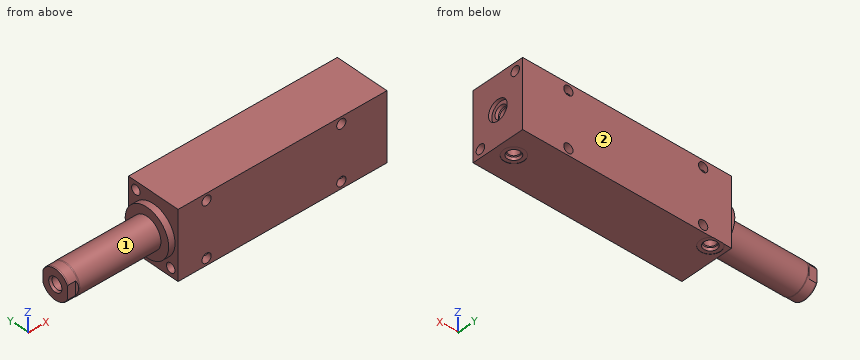
from build123d import *

# Parameters (mm, degrees)
SKETCH1_W          = 63.5
SKETCH1_H          = 50.8
EXTRUDE1_DEPTH     = 196.85
SKETCH5_R          = 22.225
EXTRUDE2_DEPTH     = 5.969
SKETCH6_W          = 14.2875
SKETCH6_H          = 86.36
CUT_EXTRUDE4_DEPTH = 30.48
HOLE1_D            = 8.7376
HOLE1_DEPTH        = 196.85
HOLE2_D            = 8.7376
HOLE2_DEPTH        = 50.8
LPATTERN1_COUNT    = 2
LPATTERN1_PITCH    = 127


with BuildPart() as part:
    # Sketch1 → Extrude1 (new body)
    with BuildSketch(Plane(origin=(0, 0, 0), x_dir=(0, 0, -1), z_dir=(1, 0, 0))):
        Rectangle(SKETCH1_W, SKETCH1_H)
    extrude(amount=EXTRUDE1_DEPTH)

    # S2D0002 → Cut-Revolve1 (revolve, cut)
    with BuildSketch(Plane(origin=(0, 17.4752, 0), x_dir=(-1, 0, 0), z_dir=(0, 1, 0)), mode=Mode.PRIVATE) as cut_revolve1_sk:
        Polygon((-18.8849, -31.496), (-22.225, -31.496), (-22.225, -31.75), (-12.7, -31.75), (-12.7, -17.526), (-17.6784, -17.526), (-17.6784, -28.279393135), (-18.342306865, -28.9433), align=None)
    revolve(cut_revolve1_sk.sketch.rotate(Axis((12.7, 17.4752, -19.13842003), (0, 0, 1)), 180), axis=Axis((12.7, 17.4752, -19.13842003), (0, 0, 1)), mode=Mode.SUBTRACT)  # turned: the seam where the file's is

    # Sketch3 → Cut-Revolve2 (revolve, cut)
    with BuildSketch(Plane(origin=(41.148, 0, -25.146), x_dir=(1, 0, 0), z_dir=(0, 1, 0))):
        Polygon((146.7993, 6.35), (150.1394, 6.35), (150.1394, 6.604), (140.6144, 6.604), (140.6144, -7.62), (145.5928, -7.62), (145.5928, 3.133393135), (146.256706865, 3.7973), align=None)
    revolve(axis=Axis((181.7624, 0, -3.189624441), (0, 0, -1)), mode=Mode.SUBTRACT)

    # Sketch4 → Cut-Revolve3 (revolve, cut)
    with BuildSketch(Plane(origin=(53.975, 0, 0), x_dir=(0, -1, 0), z_dir=(0, 0, 1)), mode=Mode.PRIVATE) as cut_revolve3_sk:
        Polygon((6.1849, 139.827), (9.525, 139.827), (9.525, 142.875), (0, 142.875), (0, 128.4732), (4.9784, 128.4732), (4.9784, 136.610393135), (5.642306865, 137.2743), align=None)
    revolve(cut_revolve3_sk.sketch.rotate(Axis((38.879609832, 0, 0), (1, 0, 0)), 270), axis=Axis((38.879609832, 0, 0), (1, 0, 0)), mode=Mode.SUBTRACT)  # turned: the seam where the file's is

    # Sketch5 → Extrude2 (add)
    with BuildSketch(Plane.ZY):
        Circle(SKETCH5_R)
    extrude(amount=EXTRUDE2_DEPTH)

    # Sketch6 → Revolve1 (revolve)
    with BuildSketch(Plane(origin=(0, 0, 0), x_dir=(0, 0, 1), z_dir=(0, -1, 0)), mode=Mode.PRIVATE) as revolve1_sk:
        with Locations((-7.14375, 49.149)):
            Rectangle(SKETCH6_W, SKETCH6_H)
    revolve(revolve1_sk.sketch.rotate(Axis((5.754582971, 0, 0), (-1, 0, 0)), 180), axis=Axis((5.754582971, 0, 0), (-1, 0, 0)))  # turned: the seam where the file's is

    # S2D0001 → Cut-Revolve4 (revolve, cut)
    with BuildSketch(Plane(origin=(-18.511260017, 3.2639, 0), x_dir=(0, 1, 0), z_dir=(0, 0, 1)), mode=Mode.PRIVATE) as cut_revolve4_sk:
        Polygon((2.286, 71.750017728), (2.286, 57.434739983), (-3.2639, 57.434739983), (-3.2639, 73.817739983), (3.4798, 73.817739983), align=None)
    revolve(cut_revolve4_sk.sketch.rotate(Axis((0, 0, 0), (-1, 0, 0)), 270), axis=Axis((0, 0, 0), (-1, 0, 0)), mode=Mode.SUBTRACT)  # turned: the seam where the file's is

    # Sketch8 → Cut-Revolve5 (revolve, cut)
    with BuildSketch(Plane(origin=(0, 0, 0), x_dir=(0, 0, -1), z_dir=(0, 1, 0)), mode=Mode.PRIVATE) as cut_revolve5_sk:
        with BuildLine():
            Line((-14.2875, 82.423), (-14.097, 83.185))
            Line((-14.097, 83.185), (-14.097, 91.313))
            ThreePointArc((-14.097, 91.313), (-13.996678675, 91.856796865), (-13.708922533, 92.329))
            Line((-13.708922533, 92.329), (-14.2875, 92.329))
            Line((-14.2875, 92.329), (-14.2875, 82.423))
        make_face()
    revolve(cut_revolve5_sk.sketch.rotate(Axis((-12.65936, 0, 0), (-1, 0, 0)), 180), axis=Axis((-12.65936, 0, 0), (-1, 0, 0)), mode=Mode.SUBTRACT)  # turned: the seam where the file's is

    # Sketch12 → Cut-Extrude4 (cut, symmetric)
    with BuildSketch(Plane(origin=(0, 0, 0), x_dir=(0, -1, 0), z_dir=(0, 0, -1))):
        Polygon((12.573, 92.329), (12.573, 84.7598), (14.097, 83.2358), (14.097, 92.329), align=None)
        Polygon((-12.573, 92.329), (-12.573, 84.7598), (-14.097, 83.2358), (-14.097, 92.329), align=None)
    extrude(amount=CUT_EXTRUDE4_DEPTH, both=True, mode=Mode.SUBTRACT)

    # Hole1
    with Locations(Plane.ZY):
        with Locations((-24.13, -17.78), (24.13, 17.78)):
            Hole(HOLE1_D / 2, depth=HOLE1_DEPTH)

    # Hole2
    with Locations(Plane(origin=(0, 25.4, 0), x_dir=(-1, 0, 0), z_dir=(0, 1, 0))):
        with Locations((-26.797, -25.4), (-26.797, 25.4)):
            hole2 = Hole(HOLE2_D / 2, depth=HOLE2_DEPTH)

    # LPattern1: Hole2 ×2
    with Locations(*[(i * LPATTERN1_PITCH, 0, 0) for i in range(1, LPATTERN1_COUNT)]):
        add(hole2, mode=Mode.SUBTRACT)


solid = part.part
For this review, take the finished solid that the model builds, in its own axes (mm). Face numbers are marked on the shaded views. A direction names the side the tool comes from. Give positions to 0.01 mm unless a question says otherwise; leave off trailing zeros. Loops run counter-clockwise (first coordinate to the right, second up) from the corner with the lowest first, then second, coordinate; pieces in that order, holes last.
Item 1: Take a section at B-B, the plane y = 0. Give the number of separate pieces and of enclosed holes in the cut face, and give its area (3 significant figures).
Item 2: Insertion check: pin 1 (10 mm diameter, centred on x = -54.5, z = 1, fed in from -Y); pin 2 (14.5 mm diameter, centred on y = 0, z = 0, fed in from +X); pin 3 (11.5 mm diameter, centred on y = -17.78, z = -24.13, fed in from -X); pin 4 (15 mm diameter, centred on y = 0, z = 3, fed in from +X). Each pin has a flat end and moves straight along its axis. Give the tip position at first contact, or say it passes through.
Item 3: Take a section at C-C, the plane z = 17. State the section outline as (x, y) points.
Item 4: Take a section at A-A, the plane x = 88. State the section outline as (y, z) points.
Item 5: Take a section at D-D, the plane x = -36.5. State the section outline as (y, z) points (1 decimal).
Item 6: Tool access review of the marked faces 1 and 2: name each direction out of +Z, -Z, +X, -X, +Y, -Y from which nothing blocks a thin tool from reaching the whole face with its end or side.
Item 7: For line 1 along X through (y, z) = (-19.5, 27.5); line 2 along Y through (x, z) = (132, -24); line 3 along X through (y, z) = (2, 22), list the stretches that pass through material, from the lowest coordinate up.
Calculated:
1. separate pieces: 1
1. enclosed holes: 4
1. area: 14,500 mm2
2. pin 1: stops at y = -14.29
2. pin 2: stops at x = 193.8
2. pin 3: stops at x = 0
2. pin 4: stops at x = 196.85
3. outline: (-5.97, -14.32) - (0, -14.32) - (0, -25.4) - (196.85, -25.4) - (196.85, 25.4) - (0, 25.4) - (0, 14.32) - (-5.97, 14.32) - close
4. outline: (-25.4, -31.75) - (25.4, -31.75) - (25.4, 31.75) - (-25.4, 31.75) - close; hole circle Ø8.74 at (-17.78, -24.13); hole circle Ø8.74 at (17.78, 24.13)
5. outline: circle Ø28.6 at (0, 0)
6. face 1: -X
6. face 2: +Z, -Z, +X, -X, +Y
7. line 1: x = 0 to 22.97, 30.63 to 149.97, 157.63 to 196.85
7. line 2: y = -25.4 to -22.15, -13.41 to 25.4
7. line 3: x = -5.97 to 24.05, 29.54 to 151.05, 156.54 to 196.85
